Read the model definition and answer for the solid it produces. Units are mm, in the model's axes. Face numbers are marked on the shaded views. A direction names the side the tool comes from. Round coordinates to 2 decimals unless told otherwise and drop trailing zeros. Write each loop counter-clockwise with the first axis right and the second up, starting at its lowest first coordinate (ties: lowest second). Pieces come first, ordered by that corner, then holes.
from build123d import *

# Parameters (mm, degrees)
SKETCH1_W           = 47.6
SKETCH1_H           = 28
BOSS_EXTRUDE1_DEPTH = 55
SKETCH3_R           = 2
CUT_EXTRUDE1_DEPTH  = 3
SKETCH4_W           = 18.116069914
SKETCH4_H           = 8.463303816
BOSS_EXTRUDE2_DEPTH = 5
BOSS_EXTRUDE4_DEPTH = 3
BOSS_EXTRUDE5_DEPTH = 3
SKETCH8_W           = 3
SKETCH8_H           = 28
BOSS_EXTRUDE7_DEPTH = 4
FILLET1_R           = 10
FILLET2_R           = 10
SKETCH9_R           = 1.530150167
CUT_EXTRUDE2_DEPTH  = 69.106093707
SKETCH10_W          = 37.6
SKETCH10_H          = 23
CUT_EXTRUDE4_DEPTH  = 40


with BuildPart() as part:
    # Sketch1 → Boss-Extrude1 (new body)
    with BuildSketch(Plane.XY):
        Rectangle(SKETCH1_W, SKETCH1_H)
    extrude(amount=BOSS_EXTRUDE1_DEPTH)

    # Sketch3 → Cut-Extrude1 (cut)
    with BuildSketch(Plane(origin=(23.8, 0, 0), x_dir=(0, 0, -1), z_dir=(1, 0, 0))):
        with Locations(Location((-6, 0, 0), (0, 0, 90))):
            Circle(SKETCH3_R)
    extrude(amount=-CUT_EXTRUDE1_DEPTH, mode=Mode.SUBTRACT)

    # Sketch4 → Boss-Extrude2 (add)
    with BuildSketch(Plane(origin=(23.8, 0, 0), x_dir=(0, 0, -1), z_dir=(1, 0, 0))):
        with Locations((-28.659392832, -9.768348092)):
            Rectangle(SKETCH4_W, SKETCH4_H)
    extrude(amount=BOSS_EXTRUDE2_DEPTH)

    # Sketch5 → Boss-Extrude4 (add)
    with BuildSketch(Plane(origin=(23.8, 0, 0), x_dir=(0, 0, -1), z_dir=(1, 0, 0))):
        with BuildLine():
            Line((-0.345576953, 3.5), (0, 3.5))
            Line((0, 3.5), (0, 8))
            Line((0, 8), (-6, 8))
            ThreePointArc((-6, 8), (-14, 0), (-6, -8))
            Line((-6, -8), (0, -8))
            Line((0, -8), (0, -3.5))
            Line((0, -3.5), (-0.345576953, -3.5))
            ThreePointArc((-0.345576953, -3.5), (-12.65, 0), (-0.345576953, 3.5))
        make_face()
    extrude(amount=BOSS_EXTRUDE4_DEPTH)

    # Sketch6 → Boss-Extrude5 (add)
    with BuildSketch(Plane.ZY.offset(23.8)):
        with BuildLine():
            Line((0, 8), (0, 5.291502622))
            ThreePointArc((0, 5.291502622), (8.828427125, 7.483314774), (14, 0))
            ThreePointArc((14, 0), (8.828427125, -7.483314774), (0, -5.291502622))
            Line((0, -5.291502622), (0, -8))
            ThreePointArc((0, -8), (10.472135955, -8.94427191), (16, 0))
            ThreePointArc((16, 0), (10.472135955, 8.94427191), (0, 8))
        make_face()
        with BuildLine():
            ThreePointArc((0, -5.291502622), (-0.657410327, -4.436089239), (-1.193747285, -3.5))
            Line((-1.193747285, -3.5), (-3.367496998, -3.5))
            ThreePointArc((-3.367496998, -3.5), (-2.006403125, -5.991452996), (0, -8))
            Line((0, -8), (0, -5.291502622))
        make_face()
        with BuildLine():
            Line((-3.367496998, 3.5), (-1.193747285, 3.5))
            ThreePointArc((-1.193747285, 3.5), (-0.657410327, 4.436089239), (0, 5.291502622))
            Line((0, 5.291502622), (0, 8))
            ThreePointArc((0, 8), (-2.006403125, 5.991452996), (-3.367496998, 3.5))
        make_face()
    extrude(amount=BOSS_EXTRUDE5_DEPTH)

    # Sketch8 → Boss-Extrude7 (add)
    with BuildSketch(Plane(origin=(0, 0, 0), x_dir=(-1, 0, 0), z_dir=(0, 0, -1))):
        with Locations((22.3, 0)):
            Rectangle(SKETCH8_W, SKETCH8_H)
    extrude(amount=BOSS_EXTRUDE7_DEPTH)

    # Fillet1
    fillet1_edges = [part.edges().sort_by_distance(p)[0] for p in [
        (-22.3, 14, -4),
        (1.5, -14, 0),
    ]]
    fillet(fillet1_edges, radius=FILLET1_R)

    # Fillet2
    fillet2_edges = [part.edges().sort_by_distance(p)[0] for p in [
        (-22.3, -14, -4),
    ]]
    fillet(fillet2_edges, radius=FILLET2_R)

    # Sketch9 → Cut-Extrude2 (cut, through all)
    with BuildSketch(Plane(origin=(0, 14, 0), x_dir=(1, 0, 0), z_dir=(0, 1, 0))):
        with Locations(Location((-8.55, -20.5, 0), (0, 0, 270))):
            Circle(SKETCH9_R)
        with Locations(Location((11.45, -20.5, 0), (0, 0, 270))):
            Circle(SKETCH9_R)
        with Locations(Location((11.45, -36.5, 0), (0, 0, 270))):
            Circle(SKETCH9_R)
        with Locations(Location((-8.55, -36.5, 0), (0, 0, 270))):
            Circle(SKETCH9_R)
    extrude(amount=-CUT_EXTRUDE2_DEPTH, mode=Mode.SUBTRACT)

    # Sketch10 → Cut-Extrude4 (cut)
    with BuildSketch(Plane.XY.offset(55)):
        with Locations((0, -2.5)):
            Rectangle(SKETCH10_W, SKETCH10_H)
    extrude(amount=-CUT_EXTRUDE4_DEPTH, mode=Mode.SUBTRACT)


solid = part.part
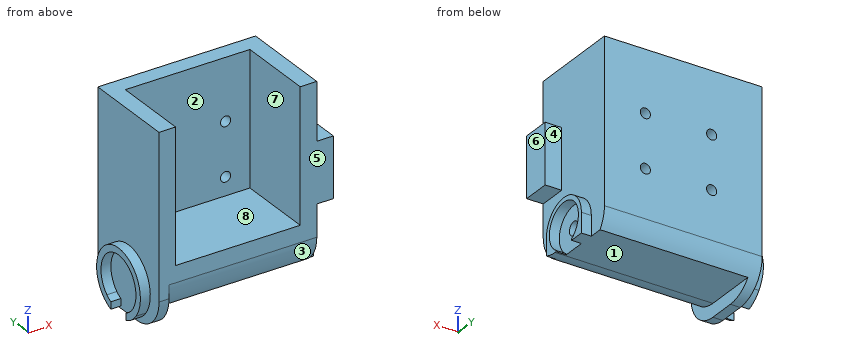
Q1. Determine the mould class of the marked faces 5, 6, 7 and 8 for opening direction X: pulls with the +X half, pulls with the -X half, needs draft (parallel to the pull), parting line crosses it, or undercut.
Verdict:
face 5: needs draft
face 6: pulls with the +X half
face 7: undercut
face 8: undercut
Q2. Section A-A (z = 36.5) is taken. Determine the outline of the cut face in (x, y), then the cut area to 3 significant figures.
Verdict:
outline: (-23.8, -14) - (-18.8, -14) - (-18.8, 9) - (-10.08, 9) - (-10.08, 14) - (-23.8, 14) - close; (-7.02, 9) - (9.92, 9) - (9.92, 14) - (-7.02, 14) - close; (12.98, 9) - (18.8, 9) - (18.8, -14) - (28.8, -14) - (28.8, -5.54) - (23.8, -5.54) - (23.8, 14) - (12.98, 14) - close
area: 480 mm2
Q3. Straight lines are drawn through the part: probe 1 along X at (y, z) = (10.45, 36.5); probe 2 along X at (y, z) = (6.5, 50); probe 3 along Z at (x, y) = (-7.5, 13). For each, find the intervals that lie inside material, in ascending order.
Verdict:
probe 1: x = -23.8 to -10.08, -7.02 to 9.92, 12.98 to 23.8
probe 2: x = -23.8 to -18.8, 18.8 to 23.8
probe 3: z = 1.64 to 19.39, 21.61 to 35.39, 37.61 to 55
Q4. Flat-ended cylindrical pins translate along their axes: pin 1 Ø0.9 at (x, z) = (25.5, 2) entering from +Y; pin 2 Ø1.1 at (x, z) = (-25, -2.5) entering from +Y; pin 3 Ø6 at (x, y) = (-21, -11) entering from -Z; pin 4 Ø3 at (x, z) = (-8.55, 36.5) entering from +Y. Find the tip coordinate at first contact, or state that the pin passes through.
Verdict:
pin 1: stops at y = 8
pin 2: stops at y = 6.07
pin 3: stops at z = -3.17
pin 4: passes through
Q5. Section C-C (y = -9) is taken. Determine the outline of the cut face in (x, z), then the cut area to 3 significant figures.
Verdict:
outline: (-26.8, 1.64) - (-23.8, 1.64) - (-23.8, -2.66) - (-20.8, -2.66) - (-20.8, 1.34) - (23.8, 1.34) - (23.8, 19.6) - (28.8, 19.6) - (28.8, 37.72) - (23.8, 37.72) - (23.8, 55) - (18.8, 55) - (18.8, 15) - (-18.8, 15) - (-18.8, 55) - (-23.8, 55) - (-23.8, 10.36) - (-26.8, 10.36) - close
area: 1,180 mm2
Q6. Section D-D (z = 27) is taken. Determine the outline of the cut face in (x, y), then the cut area to 3 significant figures.
Verdict:
outline: (-23.8, -14) - (-18.8, -14) - (-18.8, 9) - (18.8, 9) - (18.8, -14) - (28.8, -14) - (28.8, -5.54) - (23.8, -5.54) - (23.8, 14) - (-23.8, 14) - close
area: 510 mm2
Q7. Which of the six approach directions +Z, -Z, +X, -X, +Y, -Y give full straight-line access (tool end or side, diameter ignored) to the marked faces 1, 2, 3 and 4?
Verdict:
face 1: -Z, +X, +Y, -Y
face 2: +Z, -Y
face 3: -Z, +X, -Y
face 4: +Z, +X, +Y
Q8. Section B-B (x = 11.45) is taken. Determine the outline of the cut face in (y, z).
Verdict:
outline: (-14, 10) arc R10 ccw to (-4, 0) - (12, 0) arc R10 ccw to (14, 6) - (14, 18.97) - (9, 18.97) - (9, 15) - (-14, 15) - close; (9, 22.03) - (14, 22.03) - (14, 34.97) - (9, 34.97) - close; (9, 38.03) - (14, 38.03) - (14, 55) - (9, 55) - close
